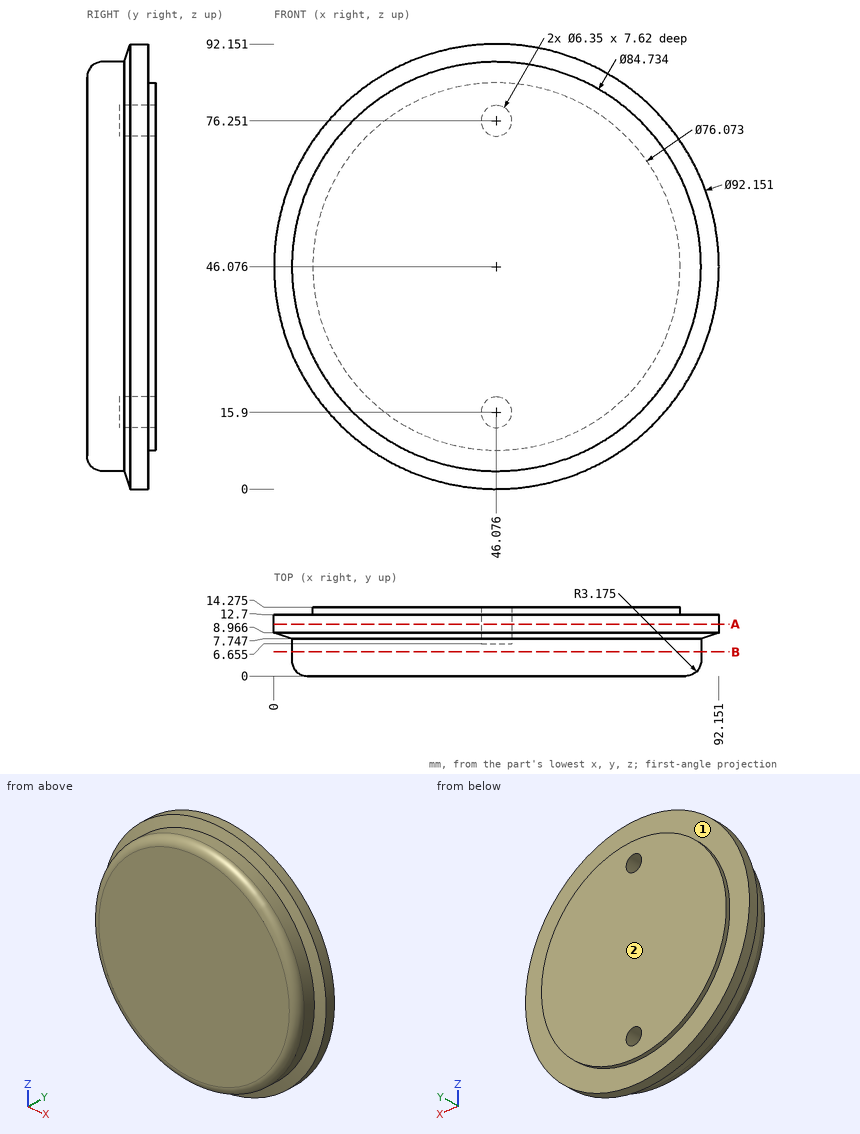
Geometry check sheet. Reference: drawing and pictorial views, mm from the part's lowest x, y, z. A direction names the side the tool comes from. Round coordinates to 2 decimals unless told otherwise and drop trailing zeros. Order: outer loops, then holes, each group sorted by start corner. A loop starts at its lowest first (then second) coordinate and runs counter-clockwise, first axis right, second up. Notation, with made-up numbers: M 51,-16 L 99,-16 A24 cw 99,8 Z; hole C 42,56.25 d2. An arc over 180 degrees is marked long. Answer in a Markdown table with one row per item.
(1) Tool access check on the marked faces 1 and 2. Record the directions out of +Z, -Z, +X, -X, +Y, -Y that give a thin tool (end or side, any length) a straight path to the whole face; none if there is none.
Responses:
| item | result |
|---|---|
| face 1 | +Y |
| face 2 | +Z, -Z, +X, -X, +Y |
(2) Sectioned sample at B-B, the plane y = 5. Record the cut outline in (x, z) (1 decimal), and give its area (3 significant figures).
Responses:
| item | result |
|---|---|
| outline | C 46.1,46.1 d84.7 |
| area | 5,640 mm² |
(3) Scan lines: probe 1 along Z at (x, y) = (48, 11.5) (1 decimal); probe 2 along Y at (x, z) = (45, 78) (1 decimal); probe 3 along X at (y, z) = (13.25, 78) (1 decimal). Record each from-to range of solid material in increasing order. Write a range as from..to.
Responses:
| item | result |
|---|---|
| probe 1 | z = 0..13.4, 18.4..73.7, 78.8..92.1 |
| probe 2 | y = 0..6.7 |
| probe 3 | x = 25.4..43.4, 48.7..66.8 |
(4) Sectioned sample at A-A, the plane y = 10.75. State how many separate pieces and enclosed holes the cut face has, and give its area (3 significant figures).
Responses:
| item | result |
|---|---|
| separate pieces | 1 |
| enclosed holes | 2 |
| area | 6,610 mm² |
(5) Go/stop test with flat-tipped pins: P1, Ø5, axis at y = 2.5, z = 50, coming from the -X side (1 decimal); P2, Ø2, axis at y = 2, z = 50, coming from the -X side; P3, Ø5.5, axis at x = 46.08, z = 15.9, coming from the -Y side; P4, Ø3, axis at x = 32.5, y = 6, coming from the +Z side (1 decimal). Record where each tip stops, or that it passes through.
Responses:
| item | result |
|---|---|
| P1 | stops at x = 3.7 |
| P2 | stops at x = 3.86 |
| P3 | stops at y = 0 |
| P4 | stops at z = 86.7 |
